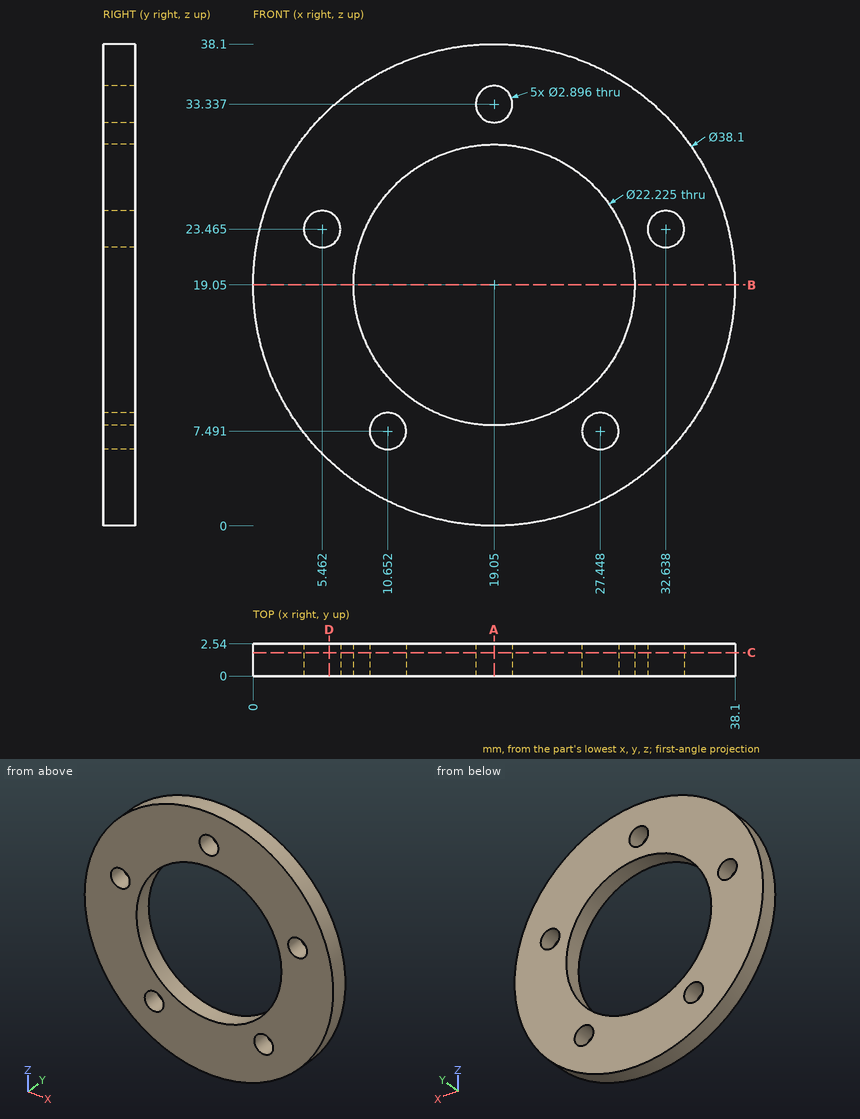
Design review of the part shown in the three views and the two pictorial views. Dimensions are in mm from the part's minimum x, y and z. Round coordinates to 2 decimals unless told otherwise and drop trailing zeros. Write each loop counter-clockwise with the first axis right and the second up, starting at its lowest first coordinate (ties: lowest second). Pieces come first, ordered by that corner, then holes. Notation, with made-up numbers: M 69,5 L 78,5 A32 cw 78,35 Z; hole C -35,46.5 d8. An arc over 180 degrees is marked long. One line per item, written item: value. Start each with the question number.
1. Take a section at B-B on z = 19.05. State the section outline as (x, y) points.
2. To check wall thickness, follow probe 1 along X at (y, z) = (2.35, 6.5) (1 decimal); probe 2 along X at (y, z) = (0.35, 19.5) (1 decimal); probe 3 along Z at (x, y) = (18, 1.15) (1 decimal). State the ranges of each line that lie inside material, in increasing order. Write a range as from..to.
3. Take a section at C-C on y = 1.85. State how many separate pieces and enclosed holes the cut face has, then the cut area to 3 significant figures.
4. Clearance check with flat-ended pins moving along their axes: P1, Ø1.5, axis at x = 26, z = 34, coming from the -Y side; P2, Ø1, axis at y = 0.5, z = 25.5, coming from the -X side; P3, Ø1.5, axis at y = 0.5, z = 7, coming from the -X side; P4, Ø1.7, axis at x = 32.64, z = 23.47, coming from the -Y side. State where each tip first meets the part, or that it passes through.
5. Take a section at A-A on x = 19.05. State the section outline as (y, z) points (1 decimal).
6. Take a section at D-D on x = 6. State the section outline as (y, z) points.
Computed:
1. outline: M 0,0 L 7.94,0 L 7.94,2.54 L 0,2.54 Z; M 30.16,0 L 38.1,0 L 38.1,2.54 L 30.16,2.54 Z
2. probe 1: x = 4.7..9.6, 11.7..26.4, 28.5..33.4
2. probe 2: x = 0..7.9, 30.2..38.1
2. probe 3: z = 0..8, 30.1..32.3, 34.3..38.1
3. separate pieces: 1
3. enclosed holes: 6
3. area: 719 mm²
4. P1: stops at y = 0
4. P2: stops at x = 0.95
4. P3: stops at x = 3.71
4. P4: passes through
5. outline: M 0,0 L 2.5,0 L 2.5,7.9 L 0,7.9 Z; M 0,30.2 L 2.5,30.2 L 2.5,31.9 L 0,31.9 Z; M 0,34.8 L 2.5,34.8 L 2.5,38.1 L 0,38.1 Z
6. outline: M 0,5.17 L 2.54,5.17 L 2.54,22.12 L 0,22.12 Z; M 0,24.81 L 2.54,24.81 L 2.54,32.93 L 0,32.93 Z
